from build123d import *

# Parameters (mm, degrees)
SKETCH1_W          = 152.4
SKETCH1_H          = 69.85
EXTRUDE1_DEPTH     = 6.35
SKETCH2_R          = 4.7625
CUT_EXTRUDE1_DEPTH = 7.35


with BuildPart() as part:
    # Sketch1 → Extrude1 (new body)
    with BuildSketch(Plane.XY):
        with Locations((749.3, 295.275)):
            Rectangle(SKETCH1_W, SKETCH1_H)
    extrude(amount=EXTRUDE1_DEPTH)

    # Sketch2 → Cut-Extrude1 (cut, through all)
    with BuildSketch(Plane.XY.offset(6.35)):
        with Locations((800.1, 270.09725)):
            Circle(SKETCH2_R)
        with Locations((704.85, 270.09725)):
            Circle(SKETCH2_R)
    extrude(amount=-CUT_EXTRUDE1_DEPTH, mode=Mode.SUBTRACT)


solid = part.part
Work out the finished part from the listing and answer in its coordinate system (mm). Coordinates: 2 decimals unless noted, no trailing zeros. Loops run counter-clockwise (first coordinate to the right, second up) from the corner with the lowest first, then second, coordinate; pieces in that order, holes last. Notation, with made-up numbers: (75, 68.25) -> (109, 68.25) arc R28 ccw to (109, 96.25) -> close; hole circle Ø3 at (-25.5, 36). An arc over 180 degrees is marked (long way). Write each question's results on one line, items separated by ' | '. Start each with the question number.
1) The mould has two halves that part along Y. Classify faces 1 (the flat face through (748, 260.35, 3)), 2 (the flat face through (825.5, 295, 3)), 3 (the cylindrical face through (804.64, 271.53, 3.22)): pulls with the +Y half, pulls with the -Y half, needs draft (parallel to the pull), parting line crosses it, or undercut.
2) Find section B-B on x = 801.5. Determine the outline of the cut face in (y, z).
3) Find section A-A on x = 704.85. Determine the outline of the cut face in (y, z), then the cut area to 3 significant figures.
4) Consider line 1 along Y through (x, z) = (704.85, 5.25); line 2 along X through (y, z) = (273.5, 3.75). Determine where each line is inside the solid, lowest interval first.
Response values:
1) face 1: pulls with the -Y half | face 2: needs draft | face 3: undercut
2) outline: (260.35, 0) -> (265.55, 0) -> (265.55, 6.35) -> (260.35, 6.35) -> close; (274.65, 0) -> (330.2, 0) -> (330.2, 6.35) -> (274.65, 6.35) -> close
3) outline: (260.35, 0) -> (265.33, 0) -> (265.33, 6.35) -> (260.35, 6.35) -> close; (274.86, 0) -> (330.2, 0) -> (330.2, 6.35) -> (274.86, 6.35) -> close | area: 383 mm^2
4) line 1: y = 260.35 to 265.33, 274.86 to 330.2 | line 2: x = 673.1 to 701.52, 708.18 to 796.77, 803.43 to 825.5
